Build history of the part. All positions in model axes, mm. A direction names the side the tool comes from. Coordinates: 2 decimals unless noted, no trailing zeros. Loops run counter-clockwise (first coordinate to the right, second up) from the corner with the lowest first, then second, coordinate; pieces in that order, holes last.
(1) Flat gauge pins, fed straight in: P1, Ø0.5, axis at y = -1.5, z = -1.5, coming from the +X side; P2, Ø0.5, axis at x = -1, y = -1.5, coming from the +Z side; P3, Ø1, axis at x = 2.5, z = 2.5, coming from the -Y side; P4, Ø2, axis at y = 11, z = -1.5, coming from the +X side. Where does each tip first touch, or does it go through?
(2) Slice it at A-A (x = 0). Give the cut face in (y, z), and give its area (3 significant figures).
(3) Slice it at B-B (z = 0). Give the cut face in (x, y), and give its area (3 significant figures).
(4) Wall check: L1, parallel to Y at x = 0, z = 0.25; L2, parallel to Y at x = 1.75, z = -0.75; L3, parallel to X at y = -0.25, z = 2. Give the ranges that are in metal, low to high.
(5) Tool access for faces 4 (the face through (1, -2.5, -1)), 5 (the face through (-1, -2, -0.5)), 6 (the face through (-2, 0, 0)): list every direction of +Z, -Z, +X, -X, +Y, -Y with a clear straight run to the whole face (end or side of a thin tool).
(6) Slice it at C-C (y = 4.5). Give the cut face in (x, z), and give its area (3 significant figures).
(7) Two-plate mould, pull along Z, no slides. Class faces 1 (the face through (-1, -2.5, -1)), 2 (the face through (0, -1, 0)), 3 (the face through (-1.71, 7.4, -0.38)): pulls with the +Z half, pulls with the -Z half, needs draft (parallel to the pull), parting line crosses it, or undercut.
from build123d import *

# Parameters (mm, degrees)
SKIZZE1_R                       = 1.75
AUFSATZ_LINEAR_AUSTRAGEN1_DEPTH = 16
SKIZZE2_R                       = 3
AUFSATZ_LINEAR_AUSTRAGEN2_DEPTH = 2.5
SCHNITT_LINEAR_AUSTRAGEN1_DEPTH = 1.5
VERRUNDUNG1_R                   = 1
FASE1_SIZE                      = 1


with BuildPart() as part:
    # Skizze1 → Aufsatz-Linear austragen1 (new body)
    with BuildSketch(Plane(origin=(0, 0, 0), x_dir=(1, 0, 0), z_dir=(0, 1, 0))):
        with Locations(Location((0, 0, 0), (0, 0, 270))):
            Circle(SKIZZE1_R)
    extrude(amount=AUFSATZ_LINEAR_AUSTRAGEN1_DEPTH)

    # Skizze2 → Aufsatz-Linear austragen2 (add)
    with BuildSketch(Plane(origin=(0, 0, 0), x_dir=(1, 0, 0), z_dir=(0, 1, 0))):
        with Locations(Location((0, 0, 0), (0, 0, 270))):
            Circle(SKIZZE2_R)
    extrude(amount=-AUFSATZ_LINEAR_AUSTRAGEN2_DEPTH)

    # Skizze3 → Schnitt-Linear austragen1 (cut)
    with BuildSketch(Plane.XZ.offset(2.5)):
        Polygon((-0.5, 2), (0.5, 2), (0.5, 0.5), (2, 0.5), (2, -0.5), (0.5, -0.5), (0.5, -2), (-0.5, -2), (-0.5, -0.5), (-2, -0.5), (-2, 0.5), (-0.5, 0.5), align=None)
    extrude(amount=-SCHNITT_LINEAR_AUSTRAGEN1_DEPTH, mode=Mode.SUBTRACT)

    # Verrundung1
    # the kernel refuses this fillet: 1 mm, written as the material it takes off along each edge
    with BuildSketch(Plane(origin=(0, -2.5, 0), x_dir=(0, 0, 1), z_dir=(-1, 0, 0))) as verrundung1_piece_1:
        with BuildLine():
            CenterArc((3 - VERRUNDUNG1_R, VERRUNDUNG1_R), VERRUNDUNG1_R, 270, 90)
            Line((3 - VERRUNDUNG1_R, 0), (3, 0))
            Line((3, 0), (3, VERRUNDUNG1_R))
        make_face()
    revolve(axis=Axis((0, -2.5, 0), (0, 1, 0)), mode=Mode.SUBTRACT)

    # Fase1
    fase1_edges = [part.edges().sort_by_distance(p)[0] for p in [
        (0, 16, -1.75),
    ]]
    chamfer(fase1_edges, length=FASE1_SIZE)


solid = part.part
Response values:
1. P1: stops at x = 2.73
1. P2: stops at z = 2.9
1. P3: passes through
1. P4: stops at x = 1.68
2. outline: (-2.5, -2) arc R1 ccw to (-1.5, -3) - (0, -3) - (0, -1.75) - (15, -1.75) - (16, -0.75) - (16, 0.75) - (15, 1.75) - (0, 1.75) - (0, 3) - (-1.5, 3) arc R1 ccw to (-2.5, 2) - (-1, 2) - (-1, -2) - close
2. area: 63.6 mm2
3. outline: (-3, -1.5) arc R1 ccw to (-2, -2.5) - (-2, -1) - (2, -1) - (2, -2.5) arc R1 ccw to (3, -1.5) - (3, 0) - (1.75, 0) - (1.75, 15) - (0.75, 16) - (-0.75, 16) - (-1.75, 15) - (-1.75, 0) - (-3, 0) - close
3. area: 63.6 mm2
4. L1: y = -1 to 16
4. L2: y = -2.5 to 0
4. L3: x = -2.24 to 2.24
5. face 4: +Z, -Z, +X, -X, -Y
5. face 5: -Y
5. face 6: +Y
6. outline: circle Ø3.5 at (0, 0)
6. area: 9.62 mm2
7. face 1: needs draft
7. face 2: undercut
7. face 3: parting line crosses it
